Work out the finished part from the listing and answer in its coordinate system (mm). A direction names the side the tool comes from. Coordinates: 2 decimals unless noted, no trailing zeros. Order: outer loops, then holes, each group sorted by start corner. A loop starts at its lowest first (then second) coordinate and runs counter-clockwise, first axis right, second up.
1. The part is cut by section C-C, the plane z = -1.25. Give the vertices of the cut face in (x, y).
2. The part is cut by section B-B, the plane y = 1. Give the vertices of the cut face in (x, z), then the cut area to 3 significant figures.
3. A tool of negligible diameter and unlimited length cuts with its end or side. For faces 1 (the cylindrical face through (3.1, 2.5, -2.5)), 2 (the cylindrical face through (2.91, 2.88, 16.17)), 3 (the flat face through (6.04, 4.83, 9.44)), 4 (the flat face through (5.145, -0.345, 9.439)), 5 (the flat face through (0.7, 2.5, 8.2)), from which of +Z, -Z, +X, -X, +Y, -Y can it reach the whole face along a straight path? Write none if from no direction.
4. The part is cut by section D-D, the plane z = 7. Give the vertices of the cut face in (x, y).
5. Determine the mould class of faces 6 (the flat face through (4.65, 5.45, 12.94)), 7 (the flat face through (3, 4, 14.2)), 8 (the cylindrical face through (1.24, 3.4, 8.45)) for opening direction Z: +Z half, -Z half, draft (parallel to the pull), parting line (faces both ways), or undercut.
6. Find the intervals of material crossed by probe 1 along Z at (x, y) = (5.75, 0.25); probe 2 along Y at (x, z) = (0.5, 5); probe 3 along Z at (x, y) = (7.5, 0.5), in increasing order.
7. Flat-ended cylindrical pins translate along their axes: pin 1 Ø1 at (x, z) = (7.5, 7) entering from -Y; pin 2 Ø4 at (x, z) = (3.5, 4) entering from +Y; pin 3 Ø2 at (y, z) = (0, 10) entering from +X; pin 4 Ø1 at (y, z) = (5, -2) entering from -X. Find the tip coordinate at first contact, or state that the pin passes through.
Autodesk Fusion 360 part; units mm, degrees
sketch "Skizze1" plane through (0, 0, 0) normal (0, 0, 1) x (1, 0, 0)
  line L0 (0, 0) -> (8.2, 0)
  line L1 (8.2, 0) -> (8.2, 5)
  line L2 (8.2, 5) -> (0, 5)
  line L3 (0, 5) -> (0, 0)
  dimension "d1" = 8.2
  dimension "d2" = 5
extrude "Extrusion1" add sketch "Skizze1" along normal blind 8.2
sketch "Skizze2" plane through (0, 0, 8.2) normal (0, 0, 1) x (-1, 0, 0)
  line L0 (0, -5) -> (0, 0)
  line L1 (0, 0) -> (-8.2, 0)
  line L2 (-8.2, 0) -> (-8.2, -5)
  line L3 (-8.2, -5) -> (0, -5)
  circle A0 centre (-4.1, -2.5) radius 3
  dimension "d5" = 6
  dimension "d6" = 2.5
  dimension "d38" = 4.1
extrude "Extrusion2" add sketch "Skizze2" along normal blind 0.5 contours L3 A0 | L1 L3 A0 | L1 A0
sketch "Skizze3" plane through (0, 0, 8.7) normal (0, 0, 1) x (-1, 0, 0)
  circle A0 centre (-4.1, -2.5) radius 3
  circle A1 centre (-4.1, -2.5) radius 2.375
  dimension "d9" = 4.75
extrude "Extrusion3" add sketch "Skizze3" along normal blind 5.5 contours A1
sketch "Skizze4" plane through (0, 0, 14.2) normal (0, 0, 1) x (-1, 0, 0)
  circle A0 centre (-4.1, -2.5) radius 2.375
  circle A1 centre (-4.1, -2.5) radius 1.25
  dimension "d12" = 2.5
sketch "Skizze5" plane through (0, 0, 0) normal (0, 0, -1) x (1, 0, 0)
  line L0 (0, 0) -> (0, -5)
  line L1 (0, -5) -> (8.2, -5)
  line L2 (8.2, -5) -> (8.2, 0)
  line L3 (8.2, 0) -> (0, 0)
  circle A0 centre (4.1, -2.5) radius 1
  circle A1 centre (6.6, -2.5) radius 1
  circle A2 centre (1.6, -2.5) radius 1
  dimension "d17" = 2
  dimension "d18" = 2.5
  dimension "d21" = 2.5
  dimension "d22" = 0
  dimension "d25" = -2.5
  dimension "d26" = 0
  dimension "d39" = 4.1
extrude "Extrusion5" add sketch "Skizze5" along normal blind 5 contours A0 | A1 | A2
sketch "Skizze6" plane through (0, 0, 8.7) normal (0, 0, 1) x (-1, 0, 0)
  circle A0 centre (-4.1, -2.5) radius 2.375
  circle A1 centre (-4.1, -2.5) radius 3
  line L0 (-7.3757, -3.7328) -> (-4.6702, -5.9532)
  line L1 (-4.6702, -5.9532) -> (-1.3945, -4.7204)
  line L2 (-1.3945, -4.7204) -> (-0.8243, -1.2672)
  line L3 (-0.8243, -1.2672) -> (-3.5298, 0.9532)
  line L4 (-3.5298, 0.9532) -> (-6.8055, -0.2796)
  line L5 (-6.8055, -0.2796) -> (-7.3757, -3.7328)
  point P0 (-4.1, -2.5)
  dimension "d29" = 3.5
extrude "Extrusion6" add sketch "Skizze6" along normal blind 1.5 contours A1 | L0 L1 L2 L3 L4 L5
extrude "Extrusion7" add sketch "Skizze4" along normal blind 4 contours A1
ref_plane "Arbeitsebene1" through (4.1, 2.5, 12.2) normal (0, 0, 1) x (-1, 0, 0)
sketch "Skizze8" plane through (4.1, 2.5, 12.2) normal (0, 0, 1) x (1, 0, 0)
  line L0 (-1.1793, 3.2572) -> (-3.4105, 0.6073)
  line L1 (-3.4105, 0.6073) -> (-2.2311, -2.6499)
  line L2 (-2.2311, -2.6499) -> (1.1793, -3.2572)
  line L3 (1.1793, -3.2572) -> (3.4105, -0.6073)
  line L4 (3.4105, -0.6073) -> (2.2311, 2.6499)
  line L5 (2.2311, 2.6499) -> (-1.1793, 3.2572)
  dimension "d40" = 3
extrude "Extrusion9" add sketch "Skizze8" along normal blind 1.5
Geometry says:
1. outline: circle Ø2 at (1.6, 2.5); circle Ø2 at (4.1, 2.5); circle Ø2 at (6.6, 2.5)
2. outline: (0, 0) - (8.2, 0) - (8.2, 8.2) - (6.7, 8.2) - (6.7, 8.7) - (6.92, 8.7) - (6.92, 10.2) - (5.94, 10.2) - (5.94, 12.2) - (6.76, 12.2) - (6.76, 13.7) - (5.94, 13.7) - (5.94, 14.2) - (2.26, 14.2) - (2.26, 13.7) - (1.45, 13.7) - (1.45, 12.2) - (2.26, 12.2) - (2.26, 10.2) - (1.15, 10.2) - (1.15, 8.7) - (1.5, 8.7) - (1.5, 8.2) - (0, 8.2) - close
2. area: 95.7 mm2
3. face 1: -Z
3. face 2: +Z
3. face 3: +X, +Y
3. face 4: +X, -Y
3. face 5: -X
4. outline: (0, 0) - (8.2, 0) - (8.2, 5) - (0, 5) - close
5. face 6: draft
5. face 7: +Z half
5. face 8: undercut
6. probe 1: z = 0 to 10.2, 12.2 to 13.7
6. probe 2: y = 0 to 5
6. probe 3: z = 0 to 8.2
7. pin 1: stops at y = 0
7. pin 2: stops at y = 5
7. pin 3: stops at x = 6.92
7. pin 4: passes through
